from build123d import *

# Parameters (mm, degrees)
F0_R     = 1.5
F1_DEPTH = 3


with BuildPart() as f1:
    # F0 (on Right) → F1 (new body)
    with BuildSketch(Plane.YZ):
        with BuildLine():
            Line((6.575, 6.060806), (-6.575, 6.060806))
            ThreePointArc((-6.575, 6.060806), (-7.282107, 5.767913), (-7.575, 5.060806))
            Line((-7.575, 5.060806), (-7.575, 0.510806))
            Line((-7.575, 0.510806), (-5.65, 0.510806))
            Line((-5.65, 0.510806), (-5.65, -25.409194))
            ThreePointArc((-5.65, -25.409194), (-5.357107, -26.1163), (-4.65, -26.409194))
            Line((-4.65, -26.409194), (4.65, -26.409194))
            ThreePointArc((4.65, -26.409194), (5.357107, -26.1163), (5.65, -25.409194))
            Line((5.65, -25.409194), (5.65, 0.510806))
            Line((5.65, 0.510806), (7.575, 0.510806))
            Line((7.575, 0.510806), (7.575, 5.060806))
            ThreePointArc((7.575, 5.060806), (7.282107, 5.767913), (6.575, 6.060806))
        make_face()
        with Locations((0, -22.409194)):
            Circle(F0_R, mode=Mode.SUBTRACT)
        with BuildLine():
            ThreePointArc((-1.5, -2.389194), (-1.207107, -1.682087), (-0.5, -1.389194))
            Line((-0.5, -1.389194), (0.5, -1.389194))
            ThreePointArc((0.5, -1.389194), (1.207107, -1.682087), (1.5, -2.389194))
            Line((1.5, -2.389194), (1.5, -11.189194))
            ThreePointArc((1.5, -11.189194), (1.207107, -11.8963), (0.5, -12.189194))
            Line((0.5, -12.189194), (-0.5, -12.189194))
            ThreePointArc((-0.5, -12.189194), (-1.207107, -11.8963), (-1.5, -11.189194))
            Line((-1.5, -11.189194), (-1.5, -2.389194))
        make_face(mode=Mode.SUBTRACT)
    extrude(amount=F1_DEPTH)


solid = f1.part
Part model, mm, in its own coordinate system. A direction names the side the tool comes from. Coordinates: 2 decimals unless noted, no trailing zeros. Loops run counter-clockwise (first coordinate to the right, second up) from the corner with the lowest first, then second, coordinate; pieces in that order, holes last. Notation, with made-up numbers: M 65.5,-5 L 102.5,-5 A14 ccw 102.5,9 Z; hole C 79.5,86.5 d7. An arc over 180 degrees is marked long. Use a Markdown table: item, result. Add a question column.
Q1. Which spindle directions (+Z, -Z, +X, -X, +Y, -Y) get a long thin tool onto all of the face, cutting with end or side? Do faces 1 (the flat face through (1, 5.65, -13)), 2 (the flat face through (1, 1.5, -7)), 3 (the flat face through (1, 0, 6.061)). Say none if no direction does.
Q2. Probe L1, parallel to Z at x = 1.6, y = 0; L2, parallel to Y at x = 2.85, z = -7.5; L3, parallel to Y at x = 0.95, z = -19.5. List the from-to ranges inside material, lowest first.
Q3. Cut at C-C (x = 1.25). Write the cut outline in (y, z) (3 decimals), and give its area (3 significant figures).
Q4. Cut at A-A (z = -3.5). Write the cut outline in (x, y).
Q5. Cut at B-B (y = 0). Write the cut outline in (x, z).
Q6. Mould opens along Y. For faces 4 (the flat face through (1, 7, 0.511)), 5 (the cylindrical face through (1.479, 1.199, -1.674)), 6 (the cylindrical face through (1.479, -5.365, -26.108)), 7 (the cylindrical face through (1.479, 5.349, -26.124)) say: +Y half, -Y half, draft (parallel to the pull), parting line (faces both ways), or undercut.
Q7. Pin check, flat tips, straight feed: P1, Ø1.5, axis at y = -0.5, z = -2, coming from the -X side; P2, Ø0.6, axis at x = 2, y = -7, coming from the -Z side; P3, Ø0.9, axis at x = 1.5, z = -18, coming from the +Y side; P4, Ø0.9, axis at x = 2, z = -16, coming from the -Y side. Stop position of each tip, or through.
Q8. Cut at D-D (z = -23.5). Write the cut outline in (x, y).
Worked out:
| question | item | result |
|---|---|---|
| 1 | face 1 | -Z, +X, -X, +Y |
| 1 | face 2 | +X, -X |
| 1 | face 3 | +Z, +X, -X, +Y, -Y |
| 2 | L1 | z = -26.41 to -23.91, -20.91 to -12.19, -1.39 to 6.06 |
| 2 | L2 | y = -5.65 to -1.5, 1.5 to 5.65 |
| 2 | L3 | y = -5.65 to 5.65 |
| 3 | outline | M -7.575,0.511 L -5.65,0.511 L -5.65,-25.409 A1 ccw -4.65,-26.409 L 4.65,-26.409 A1 ccw 5.65,-25.409 L 5.65,0.511 L 7.575,0.511 L 7.575,5.061 A1 ccw 6.575,6.061 L -6.575,6.061 A1 ccw -7.575,5.061 Z; hole C 0,-22.409 d3; hole M -1.5,-11.189 A1 ccw -0.5,-12.189 L 0.5,-12.189 A1 ccw 1.5,-11.189 L 1.5,-2.389 A1 ccw 0.5,-1.389 L -0.5,-1.389 A1 ccw -1.5,-2.389 Z |
| 3 | area | 349 mm2 |
| 4 | outline | M 0,-5.65 L 3,-5.65 L 3,-1.5 L 0,-1.5 Z; M 0,1.5 L 3,1.5 L 3,5.65 L 0,5.65 Z |
| 5 | outline | M 0,-26.41 L 3,-26.41 L 3,-23.91 L 0,-23.91 Z; M 0,-20.91 L 3,-20.91 L 3,-12.19 L 0,-12.19 Z; M 0,-1.39 L 3,-1.39 L 3,6.06 L 0,6.06 Z |
| 6 | face 4 | draft |
| 6 | face 5 | undercut |
| 6 | face 6 | -Y half |
| 6 | face 7 | +Y half |
| 7 | P1 | stops at x = 0 |
| 7 | P2 | stops at z = 0.51 |
| 7 | P3 | stops at y = 5.65 |
| 7 | P4 | stops at y = -5.65 |
| 8 | outline | M 0,-5.65 L 3,-5.65 L 3,-1.03 L 0,-1.03 Z; M 0,1.03 L 3,1.03 L 3,5.65 L 0,5.65 Z |
